from build123d import *

# Parameters (mm, degrees)
SKETCH_1_W          = 15
SKETCH_1_H          = 15
SKETCH_1_W_2        = 13
SKETCH_1_H_2        = 13
EXTRUDE_1_DEPTH     = 220
SKETCH_2_R          = 1.5
CUT_EXTRUDE_1_DEPTH = 230
SKETCH_3_R          = 4
CUT_EXTRUDE_2_DEPTH = 3
SKETCH_4_R          = 4
CUT_EXTRUDE_3_DEPTH = 3


with BuildPart() as part:
    # 草图1 → 凸台-拉伸1 (new body)
    with BuildSketch(Plane(origin=(0, 0, 0), x_dir=(0, 0, -1), z_dir=(1, 0, 0))):
        Rectangle(SKETCH_1_W, SKETCH_1_H)
        Rectangle(SKETCH_1_W_2, SKETCH_1_H_2, mode=Mode.SUBTRACT)
    extrude(amount=EXTRUDE_1_DEPTH)

    # 草图2 → 切除-拉伸1 (cut)
    with BuildSketch(Plane(origin=(0, 7.5, 0), x_dir=(1, 0, 0), z_dir=(0, 1, 0))):
        with Locations(Location((20, 0, 0), (0, 0, 270))):
            Circle(SKETCH_2_R)
        with Locations(Location((46, 0, 0), (0, 0, 270))):
            Circle(SKETCH_2_R)
        with Locations(Location((56.5, 0, 0), (0, 0, 270))):
            Circle(SKETCH_2_R)
        with Locations(Location((67, 0, 0), (0, 0, 270))):
            Circle(SKETCH_2_R)
        with Locations(Location((93, 0, 0), (0, 0, 270))):
            Circle(SKETCH_2_R)
        with Locations(Location((127, 0, 0), (0, 0, 90))):
            Circle(SKETCH_2_R)
        with Locations(Location((153, 0, 0), (0, 0, 90))):
            Circle(SKETCH_2_R)
        with Locations(Location((163.5, 0, 0), (0, 0, 90))):
            Circle(SKETCH_2_R)
        with Locations(Location((174, 0, 0), (0, 0, 90))):
            Circle(SKETCH_2_R)
        with Locations(Location((200, 0, 0), (0, 0, 90))):
            Circle(SKETCH_2_R)
    extrude(amount=-CUT_EXTRUDE_1_DEPTH, mode=Mode.SUBTRACT)

    # 草图3 → 切除-拉伸2 (cut)
    with BuildSketch(Plane(origin=(0, 7.5, 0), x_dir=(1, 0, 0), z_dir=(0, 1, 0))):
        with Locations(Location((56.5, 0, 0), (0, 0, 270))):
            Circle(SKETCH_3_R)
        with Locations(Location((163.5, 0, 0), (0, 0, 270))):
            Circle(SKETCH_3_R)
    extrude(amount=-CUT_EXTRUDE_2_DEPTH, mode=Mode.SUBTRACT)

    # 草图4 → 切除-拉伸3 (cut)
    with BuildSketch(Plane.XZ.offset(7.5)):
        with Locations(Location((20, 0, 0), (0, 0, 270))):
            Circle(SKETCH_4_R)
        with Locations(Location((46, 0, 0), (0, 0, 270))):
            Circle(SKETCH_4_R)
        with Locations(Location((67, 0, 0), (0, 0, 270))):
            Circle(SKETCH_4_R)
        with Locations(Location((93, 0, 0), (0, 0, 270))):
            Circle(SKETCH_4_R)
        with Locations(Location((127, 0, 0), (0, 0, 270))):
            Circle(SKETCH_4_R)
        with Locations(Location((153, 0, 0), (0, 0, 270))):
            Circle(SKETCH_4_R)
        with Locations(Location((174, 0, 0), (0, 0, 270))):
            Circle(SKETCH_4_R)
        with Locations(Location((200, 0, 0), (0, 0, 270))):
            Circle(SKETCH_4_R)
    extrude(amount=-CUT_EXTRUDE_3_DEPTH, mode=Mode.SUBTRACT)


solid = part.part
CAD build for the part. Positions are in the model's coordinates, mm. A direction names the side the tool comes from. Round coordinates to 2 decimals unless told otherwise and drop trailing zeros. Order: outer loops, then holes, each group sorted by start corner. A loop starts at its lowest first (then second) coordinate and runs counter-clockwise, first axis right, second up. Notation, with made-up numbers: (-29.5, 83) -> (-9.5, 83) arc R19 cw to (-9.5, 103) -> close; hole circle Ø3 at (-10, -25). An arc over 180 degrees is marked (long way). Write item = value, one per line. Start each with the question number.
(1) Cut at A-A, the plane y = -2.75. List the corners of the cut face in (x, z), then the cut area to 3 significant figures.
(2) Cut at B-B, the plane x = 115. List the corners of the cut face in (y, z), then the cut area to 3 significant figures.
(3) Pull direction Y, two halves, no side cores. Call faces 1 (the flat face through (108, 0, 7.5)), 2 (the flat face through (108, 0, -6.5)), 3 (the flat face through (108, -7.5, 0)), 4 (the flat face through (108, 6.5, 0)): released by +Y, released by -Y, zero draft, split by the parting line, or undercut.
(4) Which spindle directions (+Z, -Z, +X, -X, +Y, -Y) get a long thin tool onto all of the face, cutting with end or side? Do faces 5 (the cylindrical face through (52.595, 7.007, -0.867)), 6 (the flat face through (108, 0, 6.5)), 7 (the cylindrical face through (177.966, -7.007, 0.521)). Say none if no direction does.
(5) Pin check, flat tips, straight feed: P1, Ø6.5, axis at x = 200, z = 0, coming from the -Y side; P2, Ø2.5, axis at x = 200, z = 0, coming from the +Y side; P3, Ø7, axis at x = 56.5, z = 0, coming from the +Y side. Stop position of each tip, or through.
(6) Probe line 1 (Y direction, x = 175, z = -4.5); line 2 (Z direction, x = 93, y = 7). List the from-to ranges inside material, lowest first. Write a range as [from, to].
Model answer:
q1.outline = (0, -7.5) -> (220, -7.5) -> (220, -6.5) -> (0, -6.5) -> close; (0, 6.5) -> (220, 6.5) -> (220, 7.5) -> (0, 7.5) -> close
q1.area = 440 mm2
q2.outline = (-7.5, -7.5) -> (7.5, -7.5) -> (7.5, 7.5) -> (-7.5, 7.5) -> close; hole (-6.5, -6.5) -> (6.5, -6.5) -> (6.5, 6.5) -> (-6.5, 6.5) -> close
q2.area = 56.0 mm2
q3.face_1 = zero draft
q3.face_2 = undercut
q3.face_3 = released by -Y
q3.face_4 = undercut
q4.face_5 = +Y
q4.face_6 = +X, -X
q4.face_7 = -Y
q5.P1 = 6.5
q5.P2 = through
q5.P3 = -6.5
q6.line_1 = [-7.5, -6.5], [6.5, 7.5]
q6.line_2 = [-7.5, -1.5], [1.5, 7.5]
